from build123d import *

# Parameters (mm, degrees)
CONE001_PLACEMENT_ANGLE = 1
CYLINDER001_R           = 1.25
CYLINDER001_DEPTH       = 16
CYLINDER002_R           = 1.25
CYLINDER002_DEPTH       = 20
BOX003_W                = 5
BOX003_H                = 35
BOX003_DEPTH            = 12
BOX002_W                = 5
BOX002_H                = 35
BOX002_DEPTH            = 12
CYLINDER013_R           = 2
CYLINDER013_DEPTH       = 10
CYLINDER014_R           = 2
CYLINDER014_DEPTH       = 10
CYLINDER015_R           = 2
CYLINDER015_DEPTH       = 10
CYLINDER016_R           = 2
CYLINDER016_DEPTH       = 10
CYLINDER017_R           = 2
CYLINDER017_DEPTH       = 10
CYLINDER012_R           = 2
CYLINDER012_DEPTH       = 10
CYLINDER007_R           = 2
CYLINDER007_DEPTH       = 10
CYLINDER008_R           = 2
CYLINDER008_DEPTH       = 10
CYLINDER009_R           = 2
CYLINDER009_DEPTH       = 10
CYLINDER010_R           = 2
CYLINDER010_DEPTH       = 10
CYLINDER011_R           = 2
CYLINDER011_DEPTH       = 10
CYLINDER006_R           = 2
CYLINDER006_DEPTH       = 10
PAD013_DEPTH            = 5
BOX_W                   = 2
BOX_H                   = 10
BOX_DEPTH               = 4
CYLINDER004_R           = 2.5
CYLINDER004_DEPTH       = 4
BOX001_W                = 2
BOX001_H                = 10
BOX001_DEPTH            = 4
CYLINDER003_R           = 3.5
CYLINDER003_DEPTH       = 4
CYLINDER005_R           = 2.5
CYLINDER005_DEPTH       = 3
CYLINDER_R              = 3.5
CYLINDER_DEPTH          = 4
PAD015_DEPTH            = 10
PAD_DEPTH               = 11
PAD014_DEPTH            = 10
FILLET_R                = 0.6
FILLET001_R             = 0.6
FILLET002_R             = 0.6
FILLET003_R             = 0.6
FILLET004_R             = 0.6


with BuildPart() as cono:
    # Cone → Cone (revolve)
    with BuildSketch(Plane(origin=(-11, 61, -2), x_dir=(-1, 0, 0), z_dir=(0, 1, 0))):
        Polygon((0, 0), (3, 0), (0, 5), align=None)
    revolve(axis=Axis((-11, 61, -2), (0, 0, 1)))


with BuildPart() as cono001:
    # Cone001 → Cone001 (revolve)
    with BuildSketch(Plane.XZ):
        Polygon((0, 0), (3, 0), (0, 5), align=None)
    revolve(axis=Axis((0, 0, 0), (0, 0, 1)))


with BuildPart() as cono001_1:
    # Cone001 placement: moved
    add(cono001.part.moved(Location((-56.7, 61.2, -2))).rotate(Axis((-56.7, 61.2, -2), (0, 0, 1)), CONE001_PLACEMENT_ANGLE))


with BuildPart() as cilindro:
    # Cylinder001 → Cylinder001 (new body)
    with BuildSketch(Plane(origin=(-11, 61, -2), x_dir=(1, 0, 0), z_dir=(0, 0, 1))):
        Circle(CYLINDER001_R)
    extrude(amount=CYLINDER001_DEPTH)


with BuildPart() as cilindro001:
    # Cylinder002 → Cylinder002 (new body)
    with BuildSketch(Plane(origin=(-56.5, 61, -2), x_dir=(1, 0, 0), z_dir=(0, 0, 1))):
        Circle(CYLINDER002_R)
    extrude(amount=CYLINDER002_DEPTH)


with BuildPart() as cubo003:
    # Box003 → Box003 (new body)
    with BuildSketch(Plane(origin=(-71, 69, 2), x_dir=(1, 0, 0), z_dir=(0, 0, 1))):
        with Locations((2.5, 17.5)):
            Rectangle(BOX003_W, BOX003_H)
    extrude(amount=BOX003_DEPTH)


with BuildPart() as cubo002:
    # Box002 → Box002 (new body)
    with BuildSketch(Plane(origin=(0, 69, 2), x_dir=(1, 0, 0), z_dir=(0, 0, 1))):
        with Locations((2.5, 17.5)):
            Rectangle(BOX002_W, BOX002_H)
    extrude(amount=BOX002_DEPTH)


with BuildPart() as cilindro013:
    # Cylinder013 → Cylinder013 (new body)
    with BuildSketch(Plane(origin=(5, 73, 1), x_dir=(1, 0, 0), z_dir=(0, 0, 1))):
        Circle(CYLINDER013_R)
    extrude(amount=CYLINDER013_DEPTH)


with BuildPart() as cilindro014:
    # Cylinder014 → Cylinder014 (new body)
    with BuildSketch(Plane(origin=(5, 83, 1), x_dir=(1, 0, 0), z_dir=(0, 0, 1))):
        Circle(CYLINDER014_R)
    extrude(amount=CYLINDER014_DEPTH)


with BuildPart() as cilindro015:
    # Cylinder015 → Cylinder015 (new body)
    with BuildSketch(Plane(origin=(5, 88, 1), x_dir=(1, 0, 0), z_dir=(0, 0, 1))):
        Circle(CYLINDER015_R)
    extrude(amount=CYLINDER015_DEPTH)


with BuildPart() as cilindro016:
    # Cylinder016 → Cylinder016 (new body)
    with BuildSketch(Plane(origin=(5, 93, 1), x_dir=(1, 0, 0), z_dir=(0, 0, 1))):
        Circle(CYLINDER016_R)
    extrude(amount=CYLINDER016_DEPTH)


with BuildPart() as cilindro017:
    # Cylinder017 → Cylinder017 (new body)
    with BuildSketch(Plane(origin=(5, 98, 1), x_dir=(1, 0, 0), z_dir=(0, 0, 1))):
        Circle(CYLINDER017_R)
    extrude(amount=CYLINDER017_DEPTH)


with BuildPart() as obj1:
    # Cylinder012 → Cylinder012 (new body)
    with BuildSketch(Plane(origin=(5, 78, 1), x_dir=(1, 0, 0), z_dir=(0, 0, 1))):
        Circle(CYLINDER012_R)
    extrude(amount=CYLINDER012_DEPTH)

    # Fusion010: union Cilindro013, Cilindro014, Cilindro015, Cilindro016, Cilindro017
    add(cilindro013.part)
    add(cilindro014.part)
    add(cilindro015.part)
    add(cilindro016.part)
    add(cilindro017.part)


with BuildPart() as obj1_1:
    # Fusion010 placement: moved
    add(obj1.part.moved(Location((-76, 0, 0))))


with BuildPart() as cilindro007:
    # Cylinder007 → Cylinder007 (new body)
    with BuildSketch(Plane(origin=(5, 73, 1), x_dir=(1, 0, 0), z_dir=(0, 0, 1))):
        Circle(CYLINDER007_R)
    extrude(amount=CYLINDER007_DEPTH)


with BuildPart() as cilindro008:
    # Cylinder008 → Cylinder008 (new body)
    with BuildSketch(Plane(origin=(5, 83, 1), x_dir=(1, 0, 0), z_dir=(0, 0, 1))):
        Circle(CYLINDER008_R)
    extrude(amount=CYLINDER008_DEPTH)


with BuildPart() as cilindro009:
    # Cylinder009 → Cylinder009 (new body)
    with BuildSketch(Plane(origin=(5, 88, 1), x_dir=(1, 0, 0), z_dir=(0, 0, 1))):
        Circle(CYLINDER009_R)
    extrude(amount=CYLINDER009_DEPTH)


with BuildPart() as cilindro010:
    # Cylinder010 → Cylinder010 (new body)
    with BuildSketch(Plane(origin=(5, 93, 1), x_dir=(1, 0, 0), z_dir=(0, 0, 1))):
        Circle(CYLINDER010_R)
    extrude(amount=CYLINDER010_DEPTH)


with BuildPart() as cilindro011:
    # Cylinder011 → Cylinder011 (new body)
    with BuildSketch(Plane(origin=(5, 98, 1), x_dir=(1, 0, 0), z_dir=(0, 0, 1))):
        Circle(CYLINDER011_R)
    extrude(amount=CYLINDER011_DEPTH)


with BuildPart() as cut:
    # Cylinder006 → Cylinder006 (new body)
    with BuildSketch(Plane(origin=(5, 78, 1), x_dir=(1, 0, 0), z_dir=(0, 0, 1))):
        Circle(CYLINDER006_R)
    extrude(amount=CYLINDER006_DEPTH)

    # Fusion009: union Cilindro007, Cilindro008, Cilindro009, Cilindro010, Cilindro011
    add(cilindro007.part)
    add(cilindro008.part)
    add(cilindro009.part)
    add(cilindro010.part)
    add(cilindro011.part)

    # Fusion011: union obj1
    add(obj1_1.part)

    # Cut014: cut Cubo002
    add(cubo002.part, mode=Mode.SUBTRACT)

    # Cut: cut Cubo003
    add(cubo003.part, mode=Mode.SUBTRACT)


with BuildPart() as front_bar:
    # Sketch004 → Pad013 (new body)
    with BuildSketch(Plane.XY.offset(1)):
        Polygon((-65.5, 12), (-2, 12), (-2, 14), (-12, 14), (-12, 19), (-14, 19), (-14, 14), (-53.5, 14), (-53.5, 19), (-55.5, 19), (-55.5, 14), (-65.5, 14), align=None)
    extrude(amount=PAD013_DEPTH)


with BuildPart() as cubo:
    # Box → Box (new body)
    with BuildSketch(Plane(origin=(-5, 90, 1), x_dir=(1, 0, 0), z_dir=(0, 0, 1))):
        with Locations((1, 5)):
            Rectangle(BOX_W, BOX_H)
    extrude(amount=BOX_DEPTH)


with BuildPart() as cilindro003:
    # Cylinder004 → Cylinder004 (new body)
    with BuildSketch(Plane(origin=(-11, 61, 4), x_dir=(1, 0, 0), z_dir=(0, 0, 1))):
        Circle(CYLINDER004_R)
    extrude(amount=CYLINDER004_DEPTH)


with BuildPart() as cubo001:
    # Box001 → Box001 (new body)
    with BuildSketch(Plane(origin=(-64, 90, 1), x_dir=(1, 0, 0), z_dir=(0, 0, 1))):
        with Locations((1, 5)):
            Rectangle(BOX001_W, BOX001_H)
    extrude(amount=BOX001_DEPTH)


with BuildPart() as fusion004:
    # Cylinder003 → Cylinder003 (new body)
    with BuildSketch(Plane(origin=(-11, 61, 1), x_dir=(1, 0, 0), z_dir=(0, 0, 1))):
        Circle(CYLINDER003_R)
    extrude(amount=CYLINDER003_DEPTH)

    # Fusion003: union Cubo001
    add(cubo001.part)

    # Fusion004: union Cilindro003
    add(cilindro003.part)


with BuildPart() as cilindro005:
    # Cylinder005 → Cylinder005 (new body)
    with BuildSketch(Plane(origin=(-56.5, 61, 5), x_dir=(1, 0, 0), z_dir=(0, 0, 1))):
        Circle(CYLINDER005_R)
    extrude(amount=CYLINDER005_DEPTH)


with BuildPart() as cilindro004:
    # Cylinder → Cylinder (new body)
    with BuildSketch(Plane(origin=(-56.5, 61, 1), x_dir=(1, 0, 0), z_dir=(0, 0, 1))):
        Circle(CYLINDER_R)
    extrude(amount=CYLINDER_DEPTH)


with BuildPart() as base:
    # Sketch005 → Pad015 (new body)
    with BuildSketch(Plane(origin=(-1, 0, 2), x_dir=(1, 0, 0), z_dir=(0, 0, 1))):
        Polygon((0, 0), (-66, 0), (-66, 62), (-70, 67.82), (-70, 105), (6, 105), (6, 67.82), (0, 62), align=None)
    extrude(amount=PAD015_DEPTH)


with BuildPart() as bot_final:
    # Pad base: copy of front_bar
    add(front_bar.part)

    # Sketch → Pad (new body)
    with BuildSketch(Plane.XY):
        Polygon((0, 0), (-68, 0), (-68, 62), (-72, 67.82), (-72, 107), (6, 107), (6, 67.82), (0, 62), align=None)
    extrude(amount=PAD_DEPTH)

    # Sketch005 → Pad014 (new body)
    with BuildSketch(Plane(origin=(-1, 0, 2), x_dir=(1, 0, 0), z_dir=(0, 0, 1))):
        Polygon((0, 0), (-66, 0), (-66, 62), (-70, 67.82), (-70, 105), (6, 105), (6, 67.82), (0, 62), align=None)
    extrude(amount=PAD014_DEPTH)

    # Cut013: cut Base
    add(base.part, mode=Mode.SUBTRACT)

    # Fusion: union Cilindro004
    add(cilindro004.part)

    # Fusion012: union Cilindro005
    add(cilindro005.part)

    # Fusion013: union Fusion004
    add(fusion004.part)

    # Fusion014: union Cubo
    add(cubo.part)

    # Fusion015: union front_bar
    add(front_bar.part)

    # Fusion016: union Cut
    add(cut.part)

    # Cut016: cut Cilindro001
    add(cilindro001.part, mode=Mode.SUBTRACT)

    # Cut017: cut Cilindro
    add(cilindro.part, mode=Mode.SUBTRACT)

    # Cut018: cut Cono001
    add(cono001_1.part, mode=Mode.SUBTRACT)

    # Cut019: cut Cono
    add(cono.part, mode=Mode.SUBTRACT)

    # Fillet
    fillet_edges = [bot_final.edges().sort_by_distance(p)[0] for p in [
        (-68, 31, 0),
    ]]
    fillet(fillet_edges, radius=FILLET_R)

    # Fillet001
    fillet001_edges = [bot_final.edges().sort_by_distance(p)[0] for p in [
        (0, 31, 0),
    ]]
    fillet(fillet001_edges, radius=FILLET001_R)

    # Fillet002
    fillet002_edges = [bot_final.edges().sort_by_distance(p)[0] for p in [
        (-72, 87.41, 0),
    ]]
    fillet(fillet002_edges, radius=FILLET002_R)

    # Fillet003
    fillet003_edges = [bot_final.edges().sort_by_distance(p)[0] for p in [
        (6, 87.41, 0),
    ]]
    fillet(fillet003_edges, radius=FILLET003_R)

    # Fillet004
    fillet004_edges = [bot_final.edges().sort_by_distance(p)[0] for p in [
        (-33, 107, 0),
    ]]
    fillet(fillet004_edges, radius=FILLET004_R)


solid = bot_final.part
Geometry: final body of the model. Coordinates: model frame, mm. A direction names the side the tool comes from. Round coordinates to 2 decimals unless told otherwise and drop trailing zeros. Loops run counter-clockwise (first coordinate to the right, second up) from the corner with the lowest first, then second, coordinate; pieces in that order, holes last. Notation, with made-up numbers: (17.25, -28) - (47.25, -28) arc R29 ccw to (47.25, 9) - close; hole circle Ø11 at (40, 59.25). An arc over 180 degrees is marked (long way). Write each question's results on one line, items separated by ' | '. Start each with the question number.
1) First-contact query: P1, Ø1.5, axis at y = 55.5, z = 8.5, coming from the +X side; P2, Ø3, axis at x = -28, z = 5, coming from the -Y side; P3, Ø0.8, axis at x = 6.5, y = 89, coming from the -Z side. Flat tips, straight axial feed; report the tip coordinate or a pass-through.
2) Cut plane A-A on y = 45. Return loops of the section in (x, z), then the cut area to 3 significant figures.
3) Cut plane B-B on x = -25. Return loops of the section in (y, z).
4) Access query for faces 4 (the face through (-55.5, 17, 4)), 5 (the face through (-68, 31, 6)), 6 (the face through (-1, 31, 6)). Directions: +Z, -Z, +X, -X, +Y, -Y. A direction counts if a zero-diameter tool reaches every point of the face in a straight line with its end or side. Return the directions, or none.
5) Line query: probe 1 along X at (y, z) = (61, 4); probe 2 along Y at (x, z) = (-56.5, 2.5); probe 3 along Y at (x, z) = (-56.5, 6.5). Output: solid intervals per line, ascending. Write a range as [from, to].
6) Mould query, pull axis X, two halves, no side actions, for faces 1 (the face through (7, 73, 6)), 2 (the face through (-73, 83, 6)), 3 (the face through (-62, 95, 3)). Classes: released by +X, released by -X, zero draft, split by the parting line, or undercut.
Verdict:
1) P1: stops at x = 0 | P2: stops at y = 12 | P3: stops at z = 1
2) outline: (-68, 0.6) arc R0.6 ccw to (-67.4, 0) - (-0.6, 0) arc R0.6 ccw to (0, 0.6) - (0, 11) - (-1, 11) - (-1, 2) - (-67, 2) - (-67, 11) - (-68, 11) - close | area: 154 mm2
3) outline: (0, 0) - (106.4, 0) arc R0.6 ccw to (107, 0.6) - (107, 11) - (105, 11) - (105, 2) - (14, 2) - (14, 6) - (12, 6) - (12, 2) - (0, 2) - close
4) face 4: +Z | face 5: +Z, -Z, -X, -Y | face 6: +Z, -Y
5) probe 1: x = [-68, -67], [-60, -57.75], [-55.25, -53], [-14.5, -12.25], [-9.75, -7.5], [-1, 0] | probe 2: y = [12, 14], [57.5, 59.75], [62.25, 64.5], [105, 107] | probe 3: y = [58.5, 59.75], [62.25, 63.5], [105, 107]
6) face 1: released by +X | face 2: released by -X | face 3: undercut
